Check sheet for the modelled part. Datum: model origin and axes. Units: mm. A direction names the side the tool comes from. Round coordinates to 2 decimals unless told otherwise and drop trailing zeros. Order: outer loops, then holes, each group sorted by start corner. A loop starts at its lowest first (then second) coordinate and runs counter-clockwise, first axis right, second up.
from build123d import *

# Parameters (mm, degrees)
SKETCH1_W           = 90
SKETCH1_H           = 96
BOSS_EXTRUDE1_DEPTH = 10
BOSS_EXTRUDE2_DEPTH = 10
SKETCH3_R           = 19
SKETCH3_R_2         = 9.5
BOSS_EXTRUDE3_DEPTH = 22
RIB1_REACH          = 157.596
SKETCH4_WALL_W      = 405.846534596
SKETCH4_WALL_H      = 13


with BuildPart() as part:
    # Sketch1 → Boss-Extrude1 (new body)
    with BuildSketch(Plane(origin=(0, 0, 0), x_dir=(0, 1, 0), z_dir=(0, 0, 1))):
        Rectangle(SKETCH1_W, SKETCH1_H)
    extrude(amount=BOSS_EXTRUDE1_DEPTH)

    # Sketch2 → Boss-Extrude2 (add)
    with BuildSketch(Plane(origin=(-48, 0, 0), x_dir=(0, -1, 0), z_dir=(-1, 0, 0))):
        with BuildLine():
            Line((-45, 0), (-45, 96))
            ThreePointArc((-45, 96), (0, 141), (45, 96))
            Line((45, 96), (45, 0))
            Line((45, 0), (-45, 0))
        make_face()
    extrude(amount=-BOSS_EXTRUDE2_DEPTH)

    # Sketch3 → Boss-Extrude3 (add)
    with BuildSketch(Plane.YZ.offset(-38)):
        with Locations(Location((0, 96, 0), (0, 0, 270))):
            Circle(SKETCH3_R)
        with Locations(Location((0, 96, 0), (0, 0, 270))):
            Circle(SKETCH3_R_2, mode=Mode.SUBTRACT)
    extrude(amount=BOSS_EXTRUDE3_DEPTH)

    # Sketch4 wall → Rib1 (add, up to next)
    with BuildSketch(Plane(origin=(16, 0, 43.5), x_dir=(-0.6907323943, 0, 0.723110475283), z_dir=(0.723110475283, 0, 0.6907323943)), mode=Mode.PRIVATE) as rib1_sk1:
        Rectangle(SKETCH4_WALL_W, SKETCH4_WALL_H)
    rib1_tool1 = extrude(rib1_sk1.sketch, amount=-RIB1_REACH, mode=Mode.PRIVATE) - part.part
    add(rib1_tool1.solids().sort_by_distance((16, 0, 43.5))[0])


solid = part.part
1) Gauge pin test, flat ends, axial feed: pin 1 (21 mm diameter, centred on y = -1, z = 96.5, fed in from +X); pin 2 (6 mm diameter, centred on y = -4.5, z = 38, fed in from +X); pin 3 (3 mm diameter, centred on x = -6, y = 26.5, fed in from +Z). Record the tip position at first contact, or that the pin passes through.
2) Sectioned sample at D-D on y = 16.5. Record the cut outline in (x, z), and give its area (3 significant figures).
3) Sectioned sample at C-C on x = 34.5. Record the cut outline in (y, z).
4) Sectioned sample at A-A on x = -22. Record the cut outline in (y, z).
5) Set-up check for faces 1 (the face through (-18, 45, 9)), 2 (the face through (-16, -4, 105)), 3 (the face through (-6, 6.5, 32)), 4 (the face through (-38, 0, 96)), 5 (the face through (-43.07, 0.99, 140.99)): record each of +Z, -Z, +X, -X, +Y, -Y from which the full face is reachable in a straight line by a thin tool's end or side.
6) Scan lines: line 1 (Y direction, x = -22, z = 96); line 2 (Y direction, x = 11.5, z = 47); line 3 (X direction, y = 0, z = 128). Record each from-to range of solid material in increasing order.
7) Draft check along Z on faces 6 (the face through (-18, -45, 9)), 7 (the face through (-6, -6.5, 32)), 8 (the face through (-1, -1, 0)). Enter one of: pulls with the +Z half, pulls with the -Z half, needs draft (parallel to the pull), parting line crosses it, or undercut.
8) Sectioned sample at B-B on z = 20. Record the cut outline in (x, y).
Values found:
1. pin 1: stops at x = -16
1. pin 2: stops at x = 24.12
1. pin 3: stops at z = 10
2. outline: (-48, 0) - (48, 0) - (48, 10) - (-38, 10) - (-38, 86.58) - (-16, 86.58) - (-16, 105.42) - (-38, 105.42) - (-38, 137.87) - (-48, 137.87) - close
2. area: 2,650 mm2
3. outline: (-45, 0) - (45, 0) - (45, 10) - (6.5, 10) - (6.5, 24.13) - (-6.5, 24.13) - (-6.5, 10) - (-45, 10) - close
4. outline: (-45, 0) - (45, 0) - (45, 10) - (6.5, 10) - (6.5, 78.15) arc R19 ccw (long way) to (-6.5, 78.15) - (-6.5, 10) - (-45, 10) - close; hole circle Ø19 at (0, 96)
5. face 1: +Z, -Z, +X, -X, +Y
5. face 2: +Z, +X, +Y, -Y
5. face 3: +X, +Y
5. face 4: +X
5. face 5: +Z, +X, -X
6. line 1: y = -19 to -9.5, 9.5 to 19
6. line 2: y = -6.5 to 6.5
6. line 3: x = -48 to -38
7. face 6: needs draft
7. face 7: undercut
7. face 8: pulls with the -Z half
8. outline: (-48, -45) - (-38, -45) - (-38, -6.5) - (38.45, -6.5) - (38.45, 6.5) - (-38, 6.5) - (-38, 45) - (-48, 45) - close
